Autodesk Fusion 360 part; units mm, degrees
sketch "Sketch1" plane through (0, 0, 0) normal (0, 0, 1) x (1, 0, 0)
  line L0 (130, 0) -> (130, 50)
  line L1 (130, 50) -> (130, 70)
  line L2 (130, 70) -> (118, 70)
  line L3 (118, 70) -> (118, 50)
  line L4 (118, 50) -> (103, 50)
  line L5 (103, 50) -> (103, 70)
  line L6 (103, 70) -> (91, 70)
  line L7 (91, 70) -> (91, 50)
  line L8 (91, 50) -> (76, 50)
  line L9 (76, 50) -> (76, 70)
  line L10 (76, 70) -> (64, 70)
  line L11 (64, 70) -> (64, 50)
  line L12 (64, 50) -> (49, 50)
  line L13 (49, 50) -> (49, 70)
  line L14 (49, 70) -> (37, 70)
  line L15 (37, 70) -> (37, 50)
  line L16 (37, 50) -> (22, 50)
  line L17 (22, 50) -> (22, 70)
  line L18 (22, 70) -> (10, 70)
  line L19 (10, 70) -> (10, 50)
  line L20 (10, 50) -> (10, 0)
  line L21 (10, 0) -> (10, -20)
  line L22 (10, -20) -> (130, -20)
  line L23 (130, -20) -> (130, 0)
  dimension "d1" = 12
  dimension "d2" = 15
  dimension "d3" = 12
  dimension "d4" = 15
  dimension "d5" = 12
  dimension "d6" = 15
  dimension "d7" = 12
  dimension "d8" = 15
  dimension "d9" = 12
  dimension "d11" = 20
  dimension "d14" = 20
  dimension "d15" = 20
  dimension "d16" = 20
  dimension "d17" = 20
  dimension "d18" = 20
  dimension "d19" = 20
  dimension "d20" = 20
  dimension "d21" = 20
  dimension "d49" = 120
  dimension "d50" = 70
  dimension "d51" = 70
extrude "Extrude1" add sketch "Sketch1" along normal blind 15
hole "Hole1" at (10, 50.1961, 7.5484) direction (1, 0, 0) diameter 10 depth 120 tip angle 180
sketch "Sketch2" plane through (0, 0, 15) normal (0, 0, 1) x (-1, 0, 0)
  line L0 (-130, 20) -> (-130, -70)
  line L1 (-130, -70) -> (-118, -70)
  line L2 (-118, -70) -> (-118, -50)
  line L3 (-118, -50) -> (-103, -50)
  line L4 (-103, -50) -> (-103, -70)
  line L5 (-103, -70) -> (-91, -70)
  line L6 (-91, -70) -> (-91, -50)
  line L7 (-91, -50) -> (-76, -50)
  line L8 (-76, -50) -> (-76, -70)
  line L9 (-76, -70) -> (-64, -70)
  line L10 (-64, -70) -> (-64, -50)
  line L11 (-64, -50) -> (-49, -50)
  line L12 (-49, -50) -> (-49, -70)
  line L13 (-49, -70) -> (-37, -70)
  line L14 (-37, -70) -> (-37, -50)
  line L15 (-37, -50) -> (-22, -50)
  line L16 (-22, -50) -> (-22, -70)
  line L17 (-22, -70) -> (-10, -70)
  line L18 (-10, -70) -> (-10, 20)
  line L19 (-20, -20) -> (-120, -20)
  line L20 (-120, -20) -> (-120, -10)
  line L21 (-120, -10) -> (-20, -10)
  line L22 (-20, -10) -> (-20, -20)
  line L23 (-10, 20) -> (-130, 20)
  dimension "d28" = 100
  dimension "d29" = 10
extrude "Extrude2" add sketch "Sketch2" along normal blind 15 contours L19 L20 L21 L22
sketch "Sketch3" plane through (0, 20, 0) normal (0, 1, 0) x (-1, 0, 0)
  line L0 (-120, 15) -> (-20, 15)
  line L1 (-20, 15) -> (-20, 30)
  line L2 (-20, 30) -> (-120, 30)
  line L3 (-120, 30) -> (-120, 15)
  line L4 (-112.7366, 30) -> (-109.7366, 30)
  line L5 (-109.7366, 30) -> (-109.7366, 23)
  line L6 (-109.7366, 23) -> (-112.7366, 23)
  line L7 (-112.7366, 23) -> (-112.7366, 30)
  line L8 (-85.7366, 30) -> (-82.7366, 30)
  line L9 (-82.7366, 30) -> (-82.7366, 23)
  line L10 (-82.7366, 23) -> (-85.7366, 23)
  line L11 (-85.7366, 23) -> (-85.7366, 30)
  line L12 (-58.7366, 30) -> (-55.7366, 30)
  line L13 (-55.7366, 30) -> (-55.7366, 23)
  line L14 (-55.7366, 23) -> (-58.7366, 23)
  line L15 (-58.7366, 23) -> (-58.7366, 30)
  line L16 (-31.7366, 30) -> (-28.7366, 30)
  line L17 (-28.7366, 30) -> (-28.7366, 23)
  line L18 (-28.7366, 23) -> (-31.7366, 23)
  line L19 (-31.7366, 23) -> (-31.7366, 30)
  dimension "d32" = 7
  dimension "d33" = 3
  dimension "d34" = 7
  dimension "d35" = 3
  dimension "d36" = 7
  dimension "d37" = 3
  dimension "d38" = 7
  dimension "d39" = 3
  dimension "d40" = 24
  dimension "d41" = 24
  dimension "d42" = 24
  dimension "d43" = 7.2634
extrude "Extrude3" cut sketch "Sketch3" against normal blind 20 contours L2 L4 L5 L6 L7 | L2 L16 L17 L18 L19 | L2 L8 L9 L10 L11 | L2 L12 L13 L14 L15
sketch "Sketch4" plane through (0, 0, 15) normal (0, 0, 1) x (-1, 0, 0)
  line L0 (-20, -10) -> (-20, -20)
  line L1 (-20, -20) -> (-120, -20)
  line L2 (-120, -20) -> (-120, -10)
  line L3 (-120, -10) -> (-20, -10)
  line L4 (-130, 20) -> (-130, -70)
  line L5 (-130, -70) -> (-118, -70)
  line L6 (-118, -70) -> (-118, -50)
  line L7 (-118, -50) -> (-103, -50)
  line L8 (-103, -50) -> (-103, -70)
  line L9 (-103, -70) -> (-91, -70)
  line L10 (-91, -70) -> (-91, -50)
  line L11 (-91, -50) -> (-76, -50)
  line L12 (-76, -50) -> (-76, -70)
  line L13 (-76, -70) -> (-64, -70)
  line L14 (-64, -70) -> (-64, -50)
  line L15 (-64, -50) -> (-49, -50)
  line L16 (-49, -50) -> (-49, -70)
  line L17 (-49, -70) -> (-37, -70)
  line L18 (-37, -70) -> (-37, -50)
  line L19 (-37, -50) -> (-22, -50)
  line L20 (-22, -50) -> (-22, -70)
  line L21 (-22, -70) -> (-10, -70)
  line L22 (-10, -70) -> (-10, 20)
  line L23 (-10, 20) -> (-130, 20)
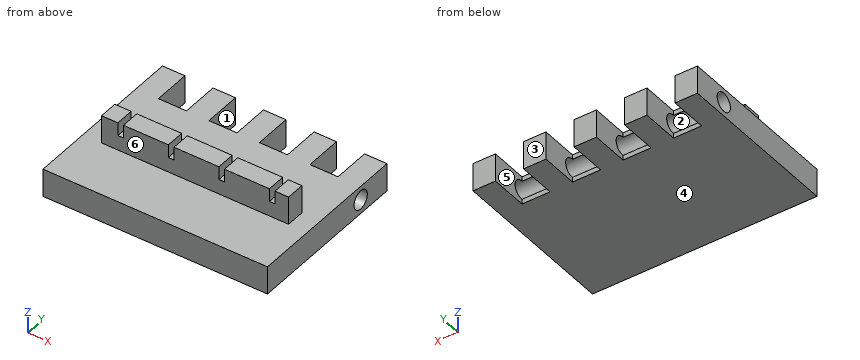
The listing builds one solid part. Answer for the finished solid, in the listing's coordinates (mm). Face numbers are marked on the shaded views. A direction names the side the tool comes from. Round coordinates to 2 decimals unless told otherwise and drop trailing zeros. Write each loop counter-clockwise with the first axis right and the second up, starting at its lowest first coordinate (ties: lowest second). Pieces come first, ordered by that corner, then holes. Notation, with made-up numbers: (16, 88) - (20, 88) arc R19 ccw to (20, 105) - close; hole circle Ø7 at (66.5, -11.75). An arc over 180 degrees is marked (long way). Use a Markdown table: item, result. Add a question column.
1. The part is cut by section B-B (z = 26). Write down the section's boundary in (x, y).
2. The part is cut by section A-A (y = 18). Write down the section's boundary in (x, z).
3. A tool of negligible diameter and unlimited length cuts with its end or side. For the marked faces 4, 5 and 6, from which of +Z, -Z, +X, -X, +Y, -Y can it reach the whole face along a straight path? Write none if from no direction.
4. The part is cut by section C-C (z = 6.5). Write down the section's boundary in (x, y).
5. Flat-ended cylindrical pins translate along their axes: P1, Ø2, axis at x = 26.5, z = 14.5, coming from the +Y side; P2, Ø4, axis at y = 19.5, z = 17.5, coming from the +X side; P3, Ø12, axis at y = 32.5, z = 22.5, coming from the +X side; P4, Ø11, axis at y = 16.5, z = 25.5, coming from the -X side. Find the tip coordinate at first contact, or state that the pin passes through.
6. The part is cut by section D-D (x = 42). Write down the section's boundary in (y, z), and give its area (3 significant figures).
7. For a pull along Y with two mould halves and no side action, classify the marked faces 1, 2 and 3 as +Y half, -Y half, draft (parallel to the pull), parting line (faces both ways), or undercut.
8. Consider line 1 (Y direction, x = 15, z = 8); line 2 (X direction, y = 58, z = 10.75); line 3 (Y direction, x = 24.5, z = 20.5). Determine where each line is inside the solid, lowest interval first.
Reported:
| question | item | result |
|---|---|---|
| 1 | outline | (20, 10) - (28.74, 10) - (28.74, 20) - (20, 20) - close; (31.74, 10) - (55.74, 10) - (55.74, 20) - (31.74, 20) - close; (58.74, 10) - (82.74, 10) - (82.74, 20) - (58.74, 20) - close; (85.74, 10) - (109.74, 10) - (109.74, 20) - (85.74, 20) - close; (112.74, 10) - (120, 10) - (120, 20) - (112.74, 20) - close |
| 2 | outline | (10, 0) - (130, 0) - (130, 15) - (120, 15) - (120, 30) - (112.74, 30) - (112.74, 23) - (109.74, 23) - (109.74, 30) - (85.74, 30) - (85.74, 23) - (82.74, 23) - (82.74, 30) - (58.74, 30) - (58.74, 23) - (55.74, 23) - (55.74, 30) - (31.74, 30) - (31.74, 23) - (28.74, 23) - (28.74, 30) - (20, 30) - (20, 15) - (10, 15) - close |
| 3 | face 4 | -Z, +X, -X, +Y, -Y |
| 3 | face 5 | +Z, -Z, +Y |
| 3 | face 6 | +Z, +X, -X, -Y |
| 4 | outline | (10, -20) - (130, -20) - (130, 45.31) - (10, 45.31) - close; (10, 55.08) - (22, 55.08) - (22, 70) - (10, 70) - close; (37, 55.08) - (49, 55.08) - (49, 70) - (37, 70) - close; (64, 55.08) - (76, 55.08) - (76, 70) - (64, 70) - close; (91, 55.08) - (103, 55.08) - (103, 70) - (91, 70) - close; (118, 55.08) - (130, 55.08) - (130, 70) - (118, 70) - close |
| 5 | P1 | y = 50 |
| 5 | P2 | x = 120 |
| 5 | P3 | through |
| 5 | P4 | x = 20 |
| 6 | outline | (-20, 0) - (70, 0) - (70, 15) - (20, 15) - (20, 30) - (10, 30) - (10, 15) - (-20, 15) - close; hole circle Ø10 at (50.2, 7.55) |
| 6 | area | 1,420 mm^2 |
| 7 | face 1 | draft |
| 7 | face 2 | undercut |
| 7 | face 3 | +Y half |
| 8 | line 1 | -20 to 45.22, 55.18 to 70 |
| 8 | line 2 | 10 to 22, 37 to 49, 64 to 76, 91 to 103, 118 to 130 |
| 8 | line 3 | 10 to 20 |
